Geometry check sheet. Reference: drawing and pictorial views, mm from the part's lowest x, y, z. Round coordinates to 2 decimals unless told otherwise and drop trailing zeros. Loops run counter-clockwise (first coordinate to the right, second up) from the corner with the lowest first, then second, coordinate; pieces in that order, holes last. Notation, with made-up numbers: (69, 51) - (97, 51) arc R17 ccw to (97, 80) - close; hole circle Ø5 at (3.25, 61.5). An arc over 180 degrees is marked (long way). Return JSON: item names as keys, results as strings.
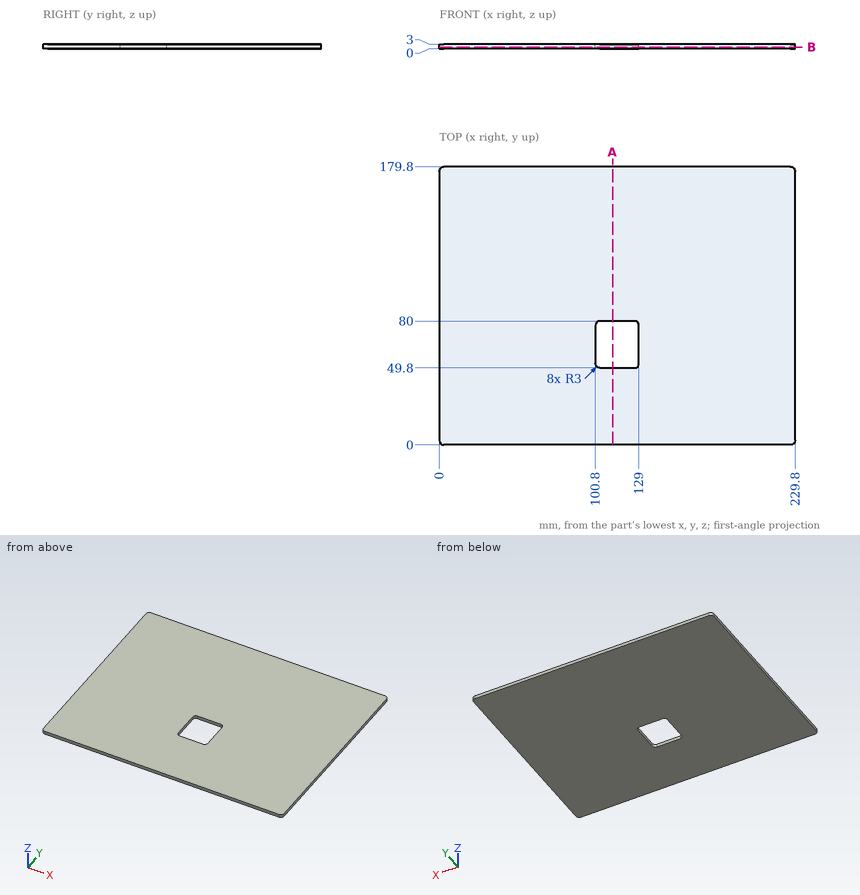
Q1. Sectioned sample at B-B (z = 1.05). Enter the section's corners in (x, y).
Answer key:
{"outline": "(0, 3) arc R3 ccw to (3, 0) - (226.8, 0) arc R3 ccw to (229.8, 3) - (229.8, 176.8) arc R3 ccw to (226.8, 179.8) - (3, 179.8) arc R3 ccw to (0, 176.8) - close; hole (100.8, 52.8) arc R3 ccw to (103.8, 49.8) - (126, 49.8) arc R3 ccw to (129, 52.8) - (129, 77) arc R3 ccw to (126, 80) - (103.8, 80) arc R3 ccw to (100.8, 77) - close"}
Q2. Depth check by flat-ended pin: P1, Ø1, axis at y = 61.5, z = 1.5, coming from the -X side. Enter the tip coordinate at first touch or a pass-through.
Answer key:
{"P1": "stops at x = 0"}
Q3. Scan lines: probe 1 along Y at (x, z) = (119, 0.3); probe 2 along X at (y, z) = (77, 2.8). Record each from-to range of solid material in increasing order. Write a range as [from, to].
Answer key:
{"probe 1": "y = [0, 49.8], [80, 179.8]", "probe 2": "x = [0, 100.8], [129, 229.8]"}
Q4. Sectioned sample at A-A (x = 112). Enter the section's corners in (y, z), plus the area to 3 significant figures.
Answer key:
{"outline": "(0, 0) - (49.8, 0) - (49.8, 3) - (0, 3) - close; (80, 0) - (179.8, 0) - (179.8, 3) - (80, 3) - close", "area": "449 mm²"}
